Autodesk Inventor part; units mm, degrees
ref_plane "Plano de trabajo1" through (0, 0, -14) normal (0, 0, 1) x (1, 0, 0)
ref_plane "YZ Plane" through (0, 0, 0) normal (1, 0, 0) x (0, 1, 0)
ref_plane "XZ Plane" through (0, 0, 0) normal (0, 1, 0) x (-1, 0, 0)
sketch "Boceto1" plane through (0, 0, 0) normal (0, 0, 1) x (1, 0, 0)
  circle A0 centre (0, 0) radius 4
  dimension "d0" = 8
extrude "Extrusión1" add sketch "Boceto1" against normal blind 28
ref_plane "Plano de trabajo1" through (0, 0, -14) normal (0, 0, 1) x (1, 0, 0)
sketch "Boceto2" plane through (0, 0, 0) normal (1, 0, 0) x (0, 1, 0)
  line L0 (0, 0) -> (0, -1.6) construction
  line L1 (0, -1.6) -> (-4, -1.6) construction
  line L2 (-4, 0) -> (-4, -28)
  line L3 (-4, -1.6) -> (-4, -2.3)
  line L4 (-4, -2.3) -> (-3.2, -2.3)
  line L5 (-3.2, -2.3) -> (-3.2, -1.6)
  line L6 (-4, -1.6) -> (-3.2, -1.6)
  dimension "d3" = 1.6
  dimension "d4" = 0.7
  dimension "d5" = 0.8
revolve "Revolución1" cut sketch "Boceto2" angle 360 about axis through (0, 0, 0) along (0, 0, -1)
mirror "Simetría1" about plane through (0, 0, -14) normal (0, 0, 1) of "Revolución1"
properties part number "12_Pasador"
The listing builds one solid part. Answer for the finished solid, in the listing's coordinates (mm). A direction names the side the tool comes from. Round coordinates to 2 decimals unless told otherwise and drop trailing zeros. Write each loop counter-clockwise with the first axis right and the second up, starting at its lowest first coordinate (ties: lowest second). Pieces come first, ordered by that corner, then holes. Notation, with made-up numbers: (28.5, -40) -> (80.5, -40) arc R19 cw to (80.5, -10) -> close; hole circle Ø3 at (70.25, 19.5). An arc over 180 degrees is marked (long way). Write item = value, one per line.
1) Straight lines are drawn through the part: line 1 along Z through (x, y) = (2.25, 3); line 2 along Y through (x, z) = (-2.25, -20.5); line 3 along Y through (x, z) = (-0.75, -5). For each, find the intervals that lie inside material, in ascending order. Write a range as [from, to].
Check values:
line_1 = [-28, -26.4], [-25.7, -2.3], [-1.6, 0]
line_2 = [-3.31, 3.31]
line_3 = [-3.93, 3.93]
2) Which of the six approach directions +Z, -Z, +X, -X, +Y, -Y give full straight-line access (tool end or side, diameter ignored) to faces 4 (the cylindrical face through (-0.867, -3.905, -13.836)), 5 (the flat face through (-3, 2, -2.3))?
Check values:
face_4 = +Z, -Z
face_5 = none
3) Section A-A on x = -2.5 is taken. Write down the section's boundary in (y, z), plus the area to 3 significant figures.
Check values:
outline = (-3.12, -28) -> (3.12, -28) -> (3.12, -26.4) -> (2, -26.4) -> (2, -25.7) -> (3.12, -25.7) -> (3.12, -2.3) -> (2, -2.3) -> (2, -1.6) -> (3.12, -1.6) -> (3.12, 0) -> (-3.12, 0) -> (-3.12, -1.6) -> (-2, -1.6) -> (-2, -2.3) -> (-3.12, -2.3) -> (-3.12, -25.7) -> (-2, -25.7) -> (-2, -26.4) -> (-3.12, -26.4) -> close
area = 172 mm²
4) Section C-C on z = -13.75 is taken. Write down the section's boundary in (x, y), plus the area to 3 significant figures.
Check values:
outline = circle Ø8 at (0, 0)
area = 50.3 mm²
5) For a pull along Z with two mould halves and no side action, classify faces 1 (the cylindrical face through (-0.867, -3.905, -0.789)), 2 (the flat face through (-3, -2, -25.7)), 3 (the flat face through (0, 0, 0)) as released by +Z, released by -Z, zero draft, split by the parting line, or undercut.
Check values:
face_1 = zero draft
face_2 = undercut
face_3 = released by +Z
6) Section B-B on y = 1.25 is taken. Write down the section's boundary in (x, z), plus the area to 3 significant figures.
Check values:
outline = (-3.8, -28) -> (3.8, -28) -> (3.8, -26.4) -> (2.95, -26.4) -> (2.95, -25.7) -> (3.8, -25.7) -> (3.8, -2.3) -> (2.95, -2.3) -> (2.95, -1.6) -> (3.8, -1.6) -> (3.8, 0) -> (-3.8, 0) -> (-3.8, -1.6) -> (-2.95, -1.6) -> (-2.95, -2.3) -> (-3.8, -2.3) -> (-3.8, -25.7) -> (-2.95, -25.7) -> (-2.95, -26.4) -> (-3.8, -26.4) -> close
area = 210 mm²
